Geometry: final body of the model. Coordinates: model frame, mm. Face numbers are marked on the shaded views. A direction names the side the tool comes from. Coordinates: 2 decimals unless noted, no trailing zeros. Loops run counter-clockwise (first coordinate to the right, second up) from the corner with the lowest first, then second, coordinate; pieces in that order, holes last. Notation, with made-up numbers: (78, -36.5) - (92, -36.5) arc R22 ccw to (92, -5.5) - close; hole circle Ø10 at (40.5, 12). An arc over 180 degrees is marked (long way). Put each result on its own line as item: value. Start each with the question number.
1) Section A-A on y = -54. Output: boundary loops of the cut face in (x, z), and give its area (3 significant figures).
2) Contact query for flat-ended pins moving along their axis: pin 1 Ø8 at (x, y) = (1, -23) entering from -Z; pin 2 Ø3.5 at (x, z) = (-11, 4) entering from +Y; pin 3 Ø2.5 at (y, z) = (-51, 6) entering from +X; pin 4 Ø4 at (y, z) = (-52, 4) entering from -X. Output: stop coordinate, or through.
3) Section C-C on z = 4. Output: boundary loops of the cut face in (x, y), and give its area (3 significant figures).
4) Section D-D on x = -11. Output: boundary loops of the cut face in (y, z) (3 decimals), and give its area (3 significant figures).
5) Material intervals for line 1 along Z through (x, y) = (-11, -60); line 2 along Y through (x, z) = (0, 5.25); line 3 along X through (y, z) = (-57, 2.75), sorted ascending. Write a range as from..to.
6) Section B-B on x = 0. Output: boundary loops of the cut face in (y, z).
7) Draft query along Y for the marked faces 1, 2, 3 and 4. Return one class per face: +Y half, -Y half, draft (parallel to the pull), parting line (faces both ways), or undercut.
8) Reachability of the marked faces 5 and 6 from +Z, -Z, +X, -X, +Y, -Y: full face, straight path, thin tool, end or side. Return the list, or none.
```python
from build123d import *

# Parameters (mm, degrees)
SKETCH_1_R          = 50
SKETCH_1_R_2        = 1.7
EXTRUDE_1_DEPTH     = 8
SKETCH_2_R          = 30.5
CUT_EXTRUDE_1_DEPTH = 8
CUT_EXTRUDE_6_DEPTH = 84
EXTRUDE_START       = -8
EXTRUDE_5_DEPTH     = 8
SKETCH_10_R         = 2.15
CUT_EXTRUDE_7_DEPTH = 8


with BuildPart() as part:
    # 草图1 → 凸台-拉伸1 (new body)
    with BuildSketch(Plane.XY):
        Circle(SKETCH_1_R)
        with Locations((0, 42.5)):
            Circle(SKETCH_1_R_2, mode=Mode.SUBTRACT)
        with Locations((30.0520382, 30.0520382)):
            Circle(SKETCH_1_R_2, mode=Mode.SUBTRACT)
        with Locations((42.5, 0)):
            Circle(SKETCH_1_R_2, mode=Mode.SUBTRACT)
        with Locations((30.0520382, -30.0520382)):
            Circle(SKETCH_1_R_2, mode=Mode.SUBTRACT)
        with Locations((0, -42.5)):
            Circle(SKETCH_1_R_2, mode=Mode.SUBTRACT)
        with Locations((-30.0520382, -30.0520382)):
            Circle(SKETCH_1_R_2, mode=Mode.SUBTRACT)
        with Locations((-42.5, 0)):
            Circle(SKETCH_1_R_2, mode=Mode.SUBTRACT)
        with Locations((-30.0520382, 30.0520382)):
            Circle(SKETCH_1_R_2, mode=Mode.SUBTRACT)
    extrude(amount=EXTRUDE_1_DEPTH)

    # 草图2 → 切除-拉伸1 (cut)
    with BuildSketch(Plane.XY.offset(8)):
        Circle(SKETCH_2_R)
    extrude(amount=-CUT_EXTRUDE_1_DEPTH, mode=Mode.SUBTRACT)

    # 草图3 → 切除-拉伸6 (cut)
    with BuildSketch(Plane.XY.offset(8)):
        with BuildLine():
            ThreePointArc((-39.400537164, -30.783074428), (-37.720132642, -17.097269866), (-24.034328132, -18.77767481))
            ThreePointArc((-24.034328132, -18.77767481), (9.7e-08, 30.5), (24.034328012, -18.777674963))
            ThreePointArc((24.034328012, -18.777674963), (37.720132595, -17.097269829), (39.400537117, -30.783074488))
            ThreePointArc((39.400537117, -30.783074488), (3.8e-08, 50), (-39.400537164, -30.783074428))
        make_face()
    extrude(amount=-CUT_EXTRUDE_6_DEPTH, mode=Mode.SUBTRACT)

    # 草图8 → 凸台-拉伸5 (add)
    with BuildSketch(Plane.XY.offset(8).offset(EXTRUDE_START)):
        with BuildLine():
            ThreePointArc((-15, -47.696960071), (-18.037363326, -46.633180507), (-21, -45.376205218))
            Line((-21, -45.376205218), (-21, -61.5))
            Line((-21, -61.5), (21, -61.5))
            Line((21, -61.5), (21, -45.376205218))
            ThreePointArc((21, -45.376205218), (18.037363326, -46.633180507), (15, -47.696960071))
            Line((15, -47.696960071), (15, -55.5))
            Line((15, -55.5), (-15, -55.5))
            Line((-15, -55.5), (-15, -47.696960071))
        make_face()
    extrude(amount=EXTRUDE_5_DEPTH)

    # 草图10 → 切除-拉伸7 (cut)
    with BuildSketch(Plane.XZ.offset(61.5)):
        with Locations((-11, 4)):
            Circle(SKETCH_10_R)
        with Locations((0, 4)):
            Circle(SKETCH_10_R)
        with Locations(Location((11, 4, 0), (0, 0, 270))):
            Circle(SKETCH_10_R)
    extrude(amount=-CUT_EXTRUDE_7_DEPTH, mode=Mode.SUBTRACT)


solid = part.part
```
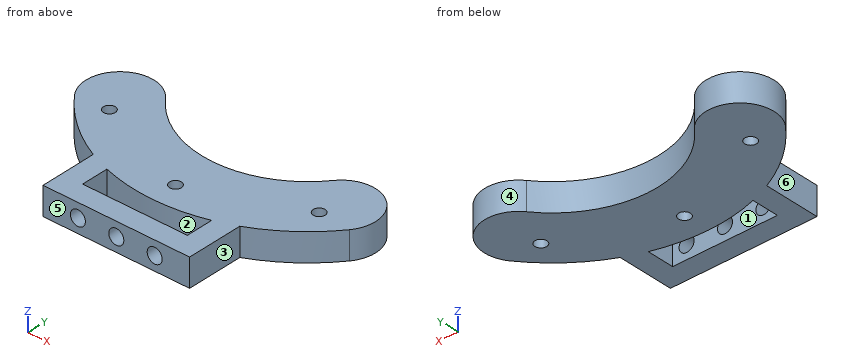
Answer block:
1. outline: (-21, 0) - (-15, 0) - (-15, 8) - (-21, 8) - close; (15, 0) - (21, 0) - (21, 8) - (15, 8) - close
1. area: 96.0 mm²
2. pin 1: passes through
2. pin 2: stops at y = -27.71
2. pin 3: stops at x = 21
2. pin 4: stops at x = -21
3. outline: (-39.4, -30.78) arc R50 ccw to (-21, -45.38) - (-21, -61.5) - (-13.15, -61.5) - (-13.15, -55.5) - (-15, -55.5) - (-15, -47.7) arc R50 ccw to (15, -47.7) - (15, -55.5) - (13.15, -55.5) - (13.15, -61.5) - (21, -61.5) - (21, -45.38) arc R50 ccw to (39.4, -30.78) arc R9.75 ccw to (24.03, -18.78) arc R30.5 cw to (-24.03, -18.78) arc R9.75 ccw to start; (-8.85, -61.5) - (-2.15, -61.5) - (-2.15, -55.5) - (-8.85, -55.5) - close; (2.15, -61.5) - (8.85, -61.5) - (8.85, -55.5) - (2.15, -55.5) - close; hole circle Ø3.4 at (-30.05, -30.05); hole circle Ø3.4 at (0, -42.5); hole circle Ø3.4 at (30.05, -30.05)
3. area: 1,980 mm²
4. outline: (-61.5, 0) - (-55.5, 0) - (-55.5, 1.85) - (-61.5, 1.85) - close; (-61.5, 6.15) - (-55.5, 6.15) - (-55.5, 8) - (-61.5, 8) - close; (-48.775, 0) - (-28.447, 0) - (-28.447, 8) - (-48.775, 8) - close
4. area: 185 mm²
5. line 1: z = 0..1.85, 6.15..8
5. line 2: y = -50..-44.2, -40.8..-30.5
5. line 3: x = -21..-12.75, -9.25..-1.75, 1.75..9.25, 12.75..21
6. outline: (-61.5, 0) - (-55.5, 0) - (-55.5, 1.85) - (-61.5, 1.85) - close; (-61.5, 6.15) - (-55.5, 6.15) - (-55.5, 8) - (-61.5, 8) - close; (-50, 0) - (-44.2, 0) - (-44.2, 8) - (-50, 8) - close; (-40.8, 0) - (-30.5, 0) - (-30.5, 8) - (-40.8, 8) - close
7. face 1: undercut
7. face 2: undercut
7. face 3: draft
7. face 4: parting line
8. face 5: +Z, -Z, +X, -X, -Y
8. face 6: +Z, -Z, -X, -Y
